For this review, take the finished solid that the model builds, in its own axes (mm). Face numbers are marked on the shaded views. A direction names the side the tool comes from. Round coordinates to 2 decimals unless told otherwise and drop trailing zeros. Order: outer loops, then holes, each group sorted by start corner. A loop starts at its lowest first (then second) coordinate and runs counter-clockwise, first axis right, second up. Notation, with made-up numbers: (19, -31.5) -> (67, -31.5) arc R32 ccw to (67, 5.5) -> close; hole circle Ø8 at (51, 21.5). An arc over 180 degrees is marked (long way). Use a Markdown table: item, result. Add a question column.
1) Consider section B-B (z = 1.75). State the section outline as (x, y) points, plus the area to 3 significant figures.
2) Consider section A-A (x = 38.1). State the section outline as (y, z) points (3 decimals), plus the area to 3 significant figures.
3) Draft analysis for pull direction Y (two halves, no side actions). For the marked faces 3, 4 and 5, state which applies: pulls with the +Y half, pulls with the -Y half, needs draft (parallel to the pull), parting line crosses it, or undercut.
4) Consider section D-D (z = 10). State the section outline as (x, y) points.
5) Consider section C-C (y = 54). State the section outline as (x, z) points (3 decimals).
6) Machinability: for the marked faces 1 and 2, which of the approach directions +Z, -Z, +X, -X, +Y, -Y give a long, thin tool a straight path to every point of the face, cutting with its end or side? Answer none if there is none.
7) Wall thickness on line 1 along X through (y, z) = (24, 2.35); line 2 along Y through (x, z) = (8, 11); line 3 along X through (y, z) = (17.5, 9): over which ranges is each line inside the solid? List them lowest first. Write a range as [from, to].
8) Clearance check with flat-ended pins moving along their axes: P1, Ø4.5, axis at x = 68.1, y = 84, coming from the -Z side; P2, Ø7, axis at x = 64.1, y = 10, coming from the +Z side. State where each tip first meets the part, or that it passes through.
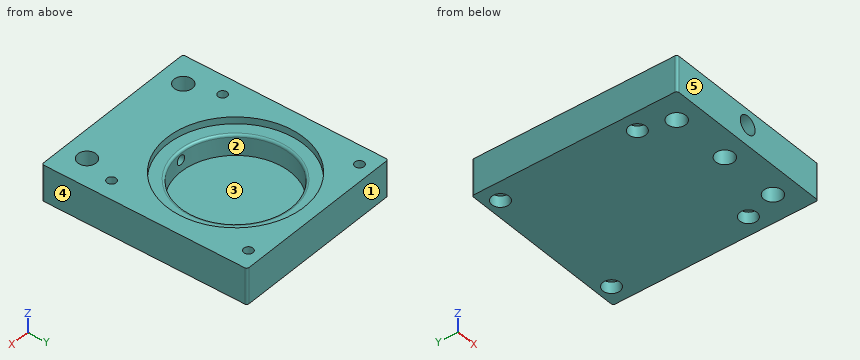
```python
from build123d import *

# Parameters (mm, degrees)
F0_W      = 76.2
F0_H      = 90
F1_DEPTH  = 15.875
F2_R      = 24
F3_DEPTH  = 12
F4_R      = 30
F4_R_2    = 24
F5_DEPTH  = 3
F6_R      = 4
F7_DEPTH  = 10
F8_R      = 4
F9_DEPTH  = 9
F12_R     = 2
F13_DEPTH = 50
F14_R     = 1
F15_R     = 2
F15_R_2   = 4
F16_DEPTH = 16
F17_R     = 3.75
F18_DEPTH = 5


with BuildPart() as f1:
    # F0 (on Top) → F1 (new body)
    with BuildSketch(Plane.XY):
        with Locations((38.1, 45)):
            Rectangle(F0_W, F0_H)
    extrude(amount=F1_DEPTH)

    # F2 (on face) → F3 (cut)
    with BuildSketch(Plane.XY.offset(15.875)):
        with Locations((38.1, 54)):
            Circle(F2_R)
    extrude(amount=-F3_DEPTH, mode=Mode.SUBTRACT)

    # F4 (on face) → F5 (cut)
    with BuildSketch(Plane.XY.offset(15.875)):
        with Locations((38.1, 54)):
            Circle(F4_R)
        with Locations((38.1, 54)):
            Circle(F4_R_2, mode=Mode.SUBTRACT)
    extrude(amount=-F5_DEPTH, mode=Mode.SUBTRACT)

    # F6 (on face) → F7 (cut)
    with BuildSketch(Plane.XZ):
        with Locations((38.1, 9)):
            Circle(F6_R)
    extrude(amount=-F7_DEPTH, mode=Mode.SUBTRACT)

    # F8 (on face) → F9 (cut)
    with BuildSketch(Plane(origin=(0, 0, 0), x_dir=(1, 0, 0), z_dir=(0, 0, -1))):
        with Locations((38.1, -10)):
            Circle(F8_R)
    extrude(amount=-F9_DEPTH, mode=Mode.SUBTRACT)

    # F10 (on face) → F11 (revolve, cut)
    with BuildSketch(Plane.XZ.offset(-10)):
        with BuildLine():
            Line((38.1, 9), (38.1, 13))
            ThreePointArc((38.1, 13), (35.2715728753, 11.8284271247), (34.1, 9))
            Line((34.1, 9), (38.1, 9))
        make_face()
    revolve(axis=Axis((38.1, 10, 9), (0, 0, -1)), mode=Mode.SUBTRACT)

    # F12 (on face) → F13 (cut)
    with BuildSketch(Plane.XZ):
        with Locations((38.1, 9)):
            Circle(F12_R)
    extrude(amount=-F13_DEPTH, mode=Mode.SUBTRACT)

    # F14
    f14_edges = [f1.edges().sort_by_distance(p)[0] for p in [
        (14.1, 54, 12.875),
        (0, 90, 7.9375),
        (0, 0, 7.9375),
        (76.2, 90, 7.9375),
        (76.2, 0, 7.9375),
    ]]
    fillet(f14_edges, radius=F14_R)

    # F15 (on face) → F16 (cut)
    with BuildSketch(Plane.XY.offset(15.875)):
        with Locations((8.1, 84)):
            Circle(F15_R)
        with Locations((68.1, 84)):
            Circle(F15_R)
        with Locations((8.1, 24)):
            Circle(F15_R)
        with Locations((68.1, 24)):
            Circle(F15_R)
        with Locations((12.1, 10)):
            Circle(F15_R_2)
        with Locations((64.1, 10)):
            Circle(F15_R_2)
    extrude(amount=-F16_DEPTH, mode=Mode.SUBTRACT)

    # F17 (on face) → F18 (cut)
    with BuildSketch(Plane(origin=(0, 0, 0), x_dir=(1, 0, 0), z_dir=(0, 0, -1))):
        with Locations((8.1, -24)):
            Circle(F17_R)
        with Locations((68.1, -24)):
            Circle(F17_R)
        with Locations((8.1, -84)):
            Circle(F17_R)
        with Locations((68.1, -84)):
            Circle(F17_R)
    extrude(amount=-F18_DEPTH, mode=Mode.SUBTRACT)


solid = f1.part
```
Results list:
| question | item | result |
|---|---|---|
| 1 | outline | (0, 1) arc R1 ccw to (1, 0) -> (75.2, 0) arc R1 ccw to (76.2, 1) -> (76.2, 89) arc R1 ccw to (75.2, 90) -> (1, 90) arc R1 ccw to (0, 89) -> close; hole circle Ø7.5 at (8.1, 24); hole circle Ø7.5 at (8.1, 84); hole circle Ø8 at (12.1, 10); hole circle Ø8 at (38.1, 10); hole circle Ø8 at (64.1, 10); hole circle Ø7.5 at (68.1, 24); hole circle Ø7.5 at (68.1, 84) |
| 1 | area | 6,530 mm2 |
| 2 | outline | (0, 0) -> (6, 0) -> (6, 5) -> (0, 5) -> close; (0, 13) -> (10, 13) arc R4 cw to (13.464, 11) -> (30, 11) -> (30, 11.875) arc R1 ccw to (29, 12.875) -> (24, 12.875) -> (24, 15.875) -> (0, 15.875) -> close; (14, 0) -> (90, 0) -> (90, 15.875) -> (84, 15.875) -> (84, 12.875) -> (79, 12.875) arc R1 ccw to (78, 11.875) -> (78, 3.875) -> (30, 3.875) -> (30, 7) -> (14, 7) -> close |
| 2 | area | 603 mm2 |
| 3 | face 3 | undercut |
| 3 | face 4 | needs draft |
| 3 | face 5 | pulls with the -Y half |
| 4 | outline | (0, 1) arc R1 ccw to (1, 0) -> (34.23, 0) -> (34.23, 10) arc R3.87 cw to (36.37, 13.46) -> (36.37, 30.06) arc R24 cw (long way) to (39.83, 30.06) -> (39.83, 13.46) arc R3.87 cw to (41.97, 10) -> (41.97, 0) -> (75.2, 0) arc R1 ccw to (76.2, 1) -> (76.2, 89) arc R1 ccw to (75.2, 90) -> (1, 90) arc R1 ccw to (0, 89) -> close; hole circle Ø4 at (8.1, 24); hole circle Ø4 at (8.1, 84); hole circle Ø8 at (12.1, 10); hole circle Ø8 at (64.1, 10); hole circle Ø4 at (68.1, 24); hole circle Ø4 at (68.1, 84) |
| 5 | outline | (0, 0) -> (76.2, 0) -> (76.2, 15.875) -> (68.1, 15.875) -> (68.1, 12.875) -> (63.1, 12.875) arc R1 ccw to (62.1, 11.875) -> (62.1, 3.875) -> (14.1, 3.875) -> (14.1, 11.875) arc R1 ccw to (13.1, 12.875) -> (8.1, 12.875) -> (8.1, 15.875) -> (0, 15.875) -> close |
| 6 | face 1 | +Z, -Z, +X, -X, +Y |
| 6 | face 2 | +Z |
| 7 | line 1 | [0, 4.35], [11.85, 64.35], [71.85, 76.2] |
| 7 | line 2 | [0, 22], [26, 82], [86, 90] |
| 7 | line 3 | [0, 36.1], [40.1, 76.2] |
| 8 | P1 | z = 5 |
| 8 | P2 | through |
